from build123d import *

# Parameters (mm, degrees)
SKETCH1_R           = 3
SKETCH1_W           = 20
SKETCH1_H           = 5
BOSS_EXTRUDE1_DEPTH = 5


with BuildPart() as part:
    # Sketch1 → Boss-Extrude1 (new body)
    with BuildSketch(Plane.XY):
        with BuildLine():
            Line((7, 0), (77, 0))
            ThreePointArc((77, 0), (79.121320344, 0.878679656), (80, 3))
            Line((80, 3), (80, 12))
            ThreePointArc((80, 12), (79.121320344, 14.121320344), (77, 15))
            Line((77, 15), (7, 15))
            ThreePointArc((7, 15), (2.050252532, 12.949747468), (0, 8))
            Line((0, 8), (0, 7))
            ThreePointArc((0, 7), (2.050252532, 2.050252532), (7, 0))
        make_face()
        with Locations((7, 7.5)):
            Circle(SKETCH1_R, mode=Mode.SUBTRACT)
        with Locations((47, 7.5)):
            Circle(SKETCH1_R, mode=Mode.SUBTRACT)
        with Locations((67, 7.75)):
            Rectangle(SKETCH1_W, SKETCH1_H, mode=Mode.SUBTRACT)
    extrude(amount=BOSS_EXTRUDE1_DEPTH)


solid = part.part
Geometry check sheet. Reference: the model listing, model coordinates, mm. A direction names the side the tool comes from. Round coordinates to 2 decimals unless told otherwise and drop trailing zeros. Loops run counter-clockwise (first coordinate to the right, second up) from the corner with the lowest first, then second, coordinate; pieces in that order, holes last. Notation, with made-up numbers: (56, 55.25) - (65, 55.25) arc R13 ccw to (65, 60.25) - close; hole circle Ø10 at (23, 68). An arc over 180 degrees is marked (long way). Answer as CSV lines item,"result".
(1) Set-up check for faces 4 (the face through (2, 2.1, 2.5)), 5 (the face through (67, 10.25, 2)): record each of +Z, -Z, +X, -X, +Y, -Y from which the full face is reachable in a straight line by a thin tool's end or side.
Output values:
face 4,"+Z, -Z, -X, -Y"
face 5,"+Z, -Z"
(2) Cross-section at C-C, the plane y = 9.25. Enter the section's corners in (x, z), and give its area (3 significant figures).
Output values:
outline,"(0.11, 0) - (4.56, 0) - (4.56, 5) - (0.11, 5) - close; (9.44, 0) - (44.56, 0) - (44.56, 5) - (9.44, 5) - close; (49.44, 0) - (57, 0) - (57, 5) - (49.44, 5) - close; (77, 0) - (80, 0) - (80, 5) - (77, 5) - close"
area,"251 mm²"
(3) Release check for a two-part mould opening along X. For faces 1 (the face through (42, 0, 2)), 2 (the face through (9.77, 6.35, 2.46)), 3 (the face through (80, 7, 2)) record: released by +X, released by -X, zero draft, split by the parting line, or undercut.
Output values:
face 1,"zero draft"
face 2,"undercut"
face 3,"released by +X"
(4) Material ranges on line 1 along Y through (x, z) = (47, 1.9); line 2 along X through (y, z) = (6.25, 2.5); line 3 along Y through (x, z) = (60.5, 4.7), recorded low to high.
Output values:
line 1,"y = 0 to 4.5, 10.5 to 15"
line 2,"x = 0.04 to 4.27, 9.73 to 44.27, 49.73 to 57, 77 to 80"
line 3,"y = 0 to 5.25, 10.25 to 15"
(5) Cross-section at D-D, the plane x = 69. Enter the section's corners in (y, z).
Output values:
outline,"(0, 0) - (5.25, 0) - (5.25, 5) - (0, 5) - close; (10.25, 0) - (15, 0) - (15, 5) - (10.25, 5) - close"
(6) Depth check by flat-ended pin: pin 1 Ø6 at (x, y) = (60.5, 6.5) entering from -Z; pin 2 Ø1.5 at (y, z) = (4.5, 3) entering from -X; pin 3 Ø5.5 at (x, y) = (47, 7.5) entering from -Z. Enter the tip coordinate at first touch or a pass-through.
Output values:
pin 1,"stops at z = 0"
pin 2,"stops at x = 0.22"
pin 3,"passes through"
(7) Cross-section at A-A, the plane x = 47. Enter the section's corners in (y, z).
Output values:
outline,"(0, 0) - (4.5, 0) - (4.5, 5) - (0, 5) - close; (10.5, 0) - (15, 0) - (15, 5) - (10.5, 5) - close"
(8) Cross-section at B-B, the plane z = 3.6. Enter the section's corners in (x, y).
Output values:
outline,"(0, 7) arc R7 ccw to (7, 0) - (77, 0) arc R3 ccw to (80, 3) - (80, 12) arc R3 ccw to (77, 15) - (7, 15) arc R7 ccw to (0, 8) - close; hole circle Ø6 at (7, 7.5); hole circle Ø6 at (47, 7.5); hole (57, 5.25) - (77, 5.25) - (77, 10.25) - (57, 10.25) - close"
